from build123d import *

# Parameters (mm, degrees)
F0_W     = 35
F0_H     = 40
F0_W_2   = 3.2
F0_H_2   = 22
F1_DEPTH = 17
F2_W     = 31
F2_H     = 13
F3_DEPTH = 35.001
F4_R     = 1.5


with BuildPart() as f1:
    # F0 (on Top) → F1 (new body)
    with BuildSketch(Plane.XY):
        Rectangle(F0_W, F0_H)
        with Locations((-10.9, 1)):
            Rectangle(F0_W_2, F0_H_2, mode=Mode.SUBTRACT)
        with Locations((10.9, 1)):
            Rectangle(F0_W_2, F0_H_2, mode=Mode.SUBTRACT)
    extrude(amount=F1_DEPTH)

    # F2 (on face) → F3 (cut, through all)
    with BuildSketch(Plane(origin=(-17.5, 0, 0), x_dir=(0, -1, 0), z_dir=(-1, 0, 0))):
        with Locations((0.5, 6.5)):
            Rectangle(F2_W, F2_H)
    extrude(amount=-F3_DEPTH, mode=Mode.SUBTRACT)

    # F4
    f4_edges = [f1.edges().sort_by_distance(p)[0] for p in [
        (-9.3, 12, 15),
        (-12.5, 12, 15),
        (-12.5, -10, 15),
        (-9.3, -10, 15),
        (9.3, -10, 15),
        (12.5, -10, 15),
        (9.3, 12, 15),
        (12.5, 12, 15),
    ]]
    fillet(f4_edges, radius=F4_R)


solid = f1.part
Here's how the part is built. I have some questions about the finished solid (model axes, mm). A direction names the side the tool comes from. Coordinates: 2 decimals unless noted, no trailing zeros. Order: outer loops, then holes, each group sorted by start corner. A loop starts at its lowest first (then second) coordinate and runs counter-clockwise, first axis right, second up. Notation, with made-up numbers: (-14.5, -2) -> (22.5, -2) arc R25 ccw to (22.5, 29) -> close; hole circle Ø7 at (89, 61.25). An arc over 180 degrees is marked (long way). Answer in a Markdown table with one row per item.
(1) I want a section at B-B on z = 6.75. List the corners of the cut face in (x, y) for me, then the cut area to 3 significant figures.
Answer key:
| item | result |
|---|---|
| outline | (-17.5, -20) -> (17.5, -20) -> (17.5, -16) -> (-17.5, -16) -> close; (-17.5, 15) -> (17.5, 15) -> (17.5, 20) -> (-17.5, 20) -> close |
| area | 315 mm^2 |
(2) Thinking about a two-plate mould opening in Y: for faces 4 (the face through (0, -16, 6)), 5 (the face through (17.5, 0, 14)), 6 (the face through (0, 20, 8)), which applies, +Y half, -Y half, draft (parallel to the pull), parting line (faces both ways), or undercut?
Answer key:
| item | result |
|---|---|
| face 4 | undercut |
| face 5 | draft |
| face 6 | +Y half |
(3) I want a section at D-D on x = -13. List the corners of the cut face in (y, z) for me, then the cut area to 3 significant figures.
Answer key:
| item | result |
|---|---|
| outline | (-20, 0) -> (-16, 0) -> (-16, 13) -> (15, 13) -> (15, 0) -> (20, 0) -> (20, 17) -> (-20, 17) -> close |
| area | 277 mm^2 |
(4) On a 3-axis mill with a long thin cutter (end or side, diameter ignored), from which of +Z, -Z, +X, -X, +Y, -Y can I reach the whole of each face in a straight line? I mean faces 1 (the face through (-9.3, 1, 15)), 2 (the face through (0, 0, 13)), 3 (the face through (0, -20, 8)). Say none if no direction works.
Answer key:
| item | result |
|---|---|
| face 1 | +Z, -Z |
| face 2 | -Z, +X, -X |
| face 3 | +Z, -Z, +X, -X, -Y |
(5) Will this pin go through, and if not, where does the flat tip stop? pin 1 Ø10 at (x, y) = (-10.5, 9) entering from -Z.
Answer key:
| item | result |
|---|---|
| pin 1 | z = 13 |
(6) I want a section at A-A on y = 1. List the corners of the cut face in (x, z) for me.
Answer key:
| item | result |
|---|---|
| outline | (-17.5, 13) -> (-12.5, 13) -> (-12.5, 17) -> (-17.5, 17) -> close; (-9.3, 13) -> (9.3, 13) -> (9.3, 17) -> (-9.3, 17) -> close; (12.5, 13) -> (17.5, 13) -> (17.5, 17) -> (12.5, 17) -> close |
(7) Please list where these lines run through material, in increasing order: probe 1 along X at (y, z) = (6, 14.25); probe 2 along Y at (x, z) = (5, 3.5); probe 3 along Z at (x, y) = (7, -2.5).
Answer key:
| item | result |
|---|---|
| probe 1 | -17.5 to -12.5, -9.3 to 9.3, 12.5 to 17.5 |
| probe 2 | -20 to -16, 15 to 20 |
| probe 3 | 13 to 17 |
(8) I want a section at C-C on z = 15.5. List the corners of the cut face in (x, y) for me, then the cut area to 3 significant figures.
Answer key:
| item | result |
|---|---|
| outline | (-17.5, -20) -> (17.5, -20) -> (17.5, 20) -> (-17.5, 20) -> close; hole (-12.5, -8.5) arc R1.5 ccw to (-11, -10) -> (-10.8, -10) arc R1.5 ccw to (-9.3, -8.5) -> (-9.3, 10.5) arc R1.5 ccw to (-10.8, 12) -> (-11, 12) arc R1.5 ccw to (-12.5, 10.5) -> close; hole (9.3, -8.5) arc R1.5 ccw to (10.8, -10) -> (11, -10) arc R1.5 ccw to (12.5, -8.5) -> (12.5, 10.5) arc R1.5 ccw to (11, 12) -> (10.8, 12) arc R1.5 ccw to (9.3, 10.5) -> close |
| area | 1,260 mm^2 |
